Source: CAD feature listing. Evaluate the final solid. Frame: model axes, mm. A direction names the side the tool comes from. Give positions to 0.01 mm unless a question says otherwise; leave off trailing zeros. Write each loop counter-clockwise with the first axis right and the second up, starting at its lowest first coordinate (ties: lowest second). Pieces come first, ordered by that corner, then holes. Notation, with made-up numbers: (80.25, -6.5) -> (100.25, -6.5) arc R29 cw to (100.25, 24.5) -> close; hole circle Ø1 at (74, -10.5). An arc over 180 degrees is marked (long way). Write item = value, one per line.
from build123d import *

# Parameters (mm, degrees)
BOSS_EXTRUDE1_DEPTH = 25
SKETCH2_R           = 2.5
CUT_EXTRUDE2_DEPTH  = 10
SKETCH3_R           = 6.260875311
BOSS_EXTRUDE2_DEPTH = 10


with BuildPart() as part:
    # Sketch1 → Boss-Extrude1 (new body)
    with BuildSketch(Plane(origin=(0, 0, 0), x_dir=(1, 0, 0), z_dir=(0, 1, 0))):
        Polygon((0, 0), (-10, 0), (-10, 24.4), (139.433967886, 24.4), (139.433967886, 0), (38.897409925, 0), (38.897409925, 20.4), (0, 20.4), align=None)
    extrude(amount=BOSS_EXTRUDE1_DEPTH)

    # Sketch2 → Cut-Extrude2 (cut)
    with BuildSketch(Plane(origin=(0, 25, 0), x_dir=(1, 0, 0), z_dir=(0, 1, 0))):
        with Locations(Location((-4.7, 15.2, 0), (0, 0, 270))):
            Circle(SKETCH2_R)
        with Locations(Location((-4.7, 5.2, 0), (0, 0, 270))):
            Circle(SKETCH2_R)
        with Locations(Location((44.9, 5.2, 0), (0, 0, 90))):
            Circle(SKETCH2_R)
        with Locations(Location((44.9, 15.2, 0), (0, 0, 90))):
            Circle(SKETCH2_R)
    extrude(amount=-CUT_EXTRUDE2_DEPTH, mode=Mode.SUBTRACT)

    # Sketch3 → Boss-Extrude2 (add)
    with BuildSketch(Plane(origin=(0, 25, 0), x_dir=(1, 0, 0), z_dir=(0, 1, 0))):
        with BuildLine():
            Line((130.655933967, 24.4), (142.775772415, 24.4))
            Line((142.775772415, 24.4), (160.225946606, 45.887947938))
            ThreePointArc((160.225946606, 45.887947938), (175.801056072, 47.503042983), (177.416151117, 31.927933517))
            Line((177.416151117, 31.927933517), (150.060915274, -1.756995769))
            Line((150.060915274, -1.756995769), (130.655933967, 0))
            Line((130.655933967, 0), (130.655933967, 24.4))
        make_face()
        with Locations(Location((168.821048861, 38.907940727, 0), (0, 0, 270))):
            Circle(SKETCH3_R, mode=Mode.SUBTRACT)
    extrude(amount=BOSS_EXTRUDE2_DEPTH)


solid = part.part
(1) Section query C-C (z = -5.2). Return loops of the section in (x, y).
Values follow:
outline = (-10, 0) -> (0, 0) -> (0, 25) -> (-2.2, 25) -> (-2.2, 15) -> (-7.2, 15) -> (-7.2, 25) -> (-10, 25) -> close; (38.9, 0) -> (139.43, 0) -> (139.43, 25) -> (155.71, 25) -> (155.71, 35) -> (130.66, 35) -> (130.66, 25) -> (47.4, 25) -> (47.4, 15) -> (42.4, 15) -> (42.4, 25) -> (38.9, 25) -> close
(2) Section query B-B (x = -4.7). Return loops of the section in (y, z), plus the area to 3 significant figures.
Values follow:
outline = (0, -24.4) -> (25, -24.4) -> (25, -17.7) -> (15, -17.7) -> (15, -12.7) -> (25, -12.7) -> (25, -7.7) -> (15, -7.7) -> (15, -2.7) -> (25, -2.7) -> (25, 0) -> (0, 0) -> close
area = 510 mm2
(3) Material intervals for line 1 (X direction, y = 23, z = -5.2); line 2 (X direction, y = 9, z = -5); line 3 (Z direction, x = 44, y = 20), sorted ascending.
Values follow:
line_1 = -10 to -7.2, -2.2 to 0, 38.9 to 42.4, 47.4 to 139.43
line_2 = -10 to 0, 38.9 to 139.43
line_3 = -24.4 to -17.53, -12.87 to -7.53, -2.87 to 0
(4) Access query for faces 1 (the face through (-5, 15, -5)), 2 (the face through (139.434, 12, -12)), 3 (the face through (163.93, 29.93, -15.32)), 4 (the face through (0, 12, -10)). Directions: +Z, -Z, +X, -X, +Y, -Y. A direction counts if a zero-diameter tool reaches every point of the face in a straight line with its end or side. Return the directions, or none.
Values follow:
face_1 = +Y
face_2 = +Z, -Z, +X, -Y
face_3 = +Z, +X, +Y, -Y
face_4 = +Z, +Y, -Y
(5) Section query D-D (y = 3). Return loops of the section in (x, z), plus the area to 3 significant figures.
Values follow:
outline = (-10, -24.4) -> (139.43, -24.4) -> (139.43, 0) -> (38.9, 0) -> (38.9, -20.4) -> (0, -20.4) -> (0, 0) -> (-10, 0) -> close
area = 2,850 mm2
(6) Pull-direction query (Z, two-part tool) for faces 5 (the face through (47.34, 20.07, -14.66)), 6 (the face through (20, 12, -20.4)), 7 (the face through (151.379, 29.93, -34.994)), 8 (the face through (-5, 15, -15)); classes: pulls with the +Z half, pulls with the -Z half, needs draft (parallel to the pull), parting line crosses it, or undercut.
Values follow:
face_5 = undercut
face_6 = pulls with the +Z half
face_7 = pulls with the -Z half
face_8 = undercut
(7) Section query A-A (y = 21). Return loops of the section in (x, z).
Values follow:
outline = (-10, -24.4) -> (139.43, -24.4) -> (139.43, 0) -> (38.9, 0) -> (38.9, -20.4) -> (0, -20.4) -> (0, 0) -> (-10, 0) -> close; hole circle Ø5 at (-4.7, -15.2); hole circle Ø5 at (-4.7, -5.2); hole circle Ø5 at (44.9, -15.2); hole circle Ø5 at (44.9, -5.2)
(8) First-contact query: pin 1 (4 mm diameter, centred on x = 45, z = -14.5, fed in from +Y); pin 2 (4 mm diameter, centred on x = 96, y = 20.5, fed in from +Z); pin 3 (1 mm diameter, centred on x = 96, y = 14.5, fed in from -Z). Flat tips, straight axial feed; report the tip coordinate or a pass-through.
Values follow:
pin_1 = 25
pin_2 = 0
pin_3 = -24.4
